from build123d import *

# Parameters (mm, degrees)
BOSS_EXTRUDE1_DEPTH   = 15
CUT_EXTRUDE1_DEPTH    = 30
SKETCH5_W             = 14
SKETCH5_H             = 36
CUT_EXTRUDE2_DEPTH    = 3
SKETCH7_R             = 1.5
CUT_EXTRUDE3_DEPTH    = 90
MIRROR1_START         = -4
MIRROR1_DEPTH         = 9
MIRROR1_START_2       = 56
MIRROR1_2_OUTLINE_W   = 60
MIRROR1_2_OUTLINE_H   = 30
MIRROR1_2_OUTLINE_W_2 = 36
MIRROR1_2_OUTLINE_H_2 = 14
MIRROR1_2_DEPTH       = 3
MIRROR1_START_3       = 59
MIRROR1_3_OUTLINE_W   = 36
MIRROR1_3_OUTLINE_H   = 14
MIRROR1_3_DEPTH       = 2
MIRROR1_4_DEPTH       = 9
MIRROR1_START_4       = 51
MIRROR1_5_DEPTH       = 4.358898944
MIRROR1_START_5       = 22.5000001
MIRROR1_6_DEPTH       = 28.4999999
MIRROR1_START_6       = -15
MIRROR1_7_OUTLINE_W   = 2
MIRROR1_7_OUTLINE_H   = 2
MIRROR1_7_DEPTH       = 30
MIRROR1_8_OUTLINE_W   = 2
MIRROR1_8_OUTLINE_H   = 36
MIRROR1_8_DEPTH       = 8
MIRROR1_START_7       = 7
MIRROR1_9_OUTLINE_W   = 2
MIRROR1_9_OUTLINE_H   = 36
MIRROR1_9_DEPTH       = 8
MIRROR1_START_8       = -6
MIRROR1_10_OUTLINE_R  = 1.5
MIRROR1_10_DEPTH      = 3
CUT_EXTRUDE5_START    = -70
CUT_EXTRUDE5_DEPTH    = 70
BOSS_EXTRUDE2_START   = -28
BOSS_EXTRUDE2_DEPTH   = 26
FILLET1_R             = 10
FILLET2_R             = 4
FILLET3_R             = 3
SKETCH9_R             = 6
CUT_EXTRUDE6_DEPTH    = 83


with BuildPart() as part:
    # Sketch1 → Boss-Extrude1 (new, symmetric)
    with BuildSketch(Plane.XY):
        with BuildLine():
            Line((5, 0), (60, 0))
            Line((60, 0), (60, -5))
            Line((60, -5), (5, -5))
            ThreePointArc((5, -5), (-2.071067812, -2.071067812), (-5, 5))
            Line((-5, 5), (-5, 60))
            Line((-5, 60), (0, 60))
            Line((0, 60), (0, 5))
            ThreePointArc((0, 5), (1.464466094, 1.464466094), (5, 0))
        make_face()
    extrude(amount=BOSS_EXTRUDE1_DEPTH, both=True)

    # Cut-Sweep1: sweep along a path in Sketch3
    with BuildLine(Plane(origin=(0, 0, 0), x_dir=(1, 0, 0), z_dir=(0, 1, 0))) as cut_sweep1_path:
        Line((60, 0), (5, 0))
    # Sketch2 → Cut-Sweep1 (sweep, cut)
    with BuildSketch(Plane(origin=(60, 0, 0), x_dir=(0, 0, -1), z_dir=(1, 0, 0))):
        Polygon((-11.5, 0), (-11.5, -1), (-13, -1), (-13, -4), (13, -4), (13, -1), (11.5, -1), (11.5, 0), align=None)
    sweep(path=cut_sweep1_path.line, mode=Mode.SUBTRACT)

    # Sketch4 → Cut-Extrude1 (cut)
    with BuildSketch(Plane(origin=(0, 0, 0), x_dir=(0, 0, -1), z_dir=(1, 0, 0))):
        with BuildLine():
            Line((1.5, 55), (1.5, 25))
            ThreePointArc((1.5, 25), (0, 23.5), (-1.5, 25))
            Line((-1.5, 25), (-1.5, 55))
            ThreePointArc((-1.5, 55), (0, 56.5), (1.5, 55))
        make_face()
    extrude(amount=-CUT_EXTRUDE1_DEPTH, mode=Mode.SUBTRACT)

    # Sketch5 → Cut-Extrude2 (cut)
    with BuildSketch(Plane(origin=(0, 0, 0), x_dir=(0, 0, -1), z_dir=(1, 0, 0))):
        with Locations((0, 40)):
            Rectangle(SKETCH5_W, SKETCH5_H)
    extrude(amount=-CUT_EXTRUDE2_DEPTH, mode=Mode.SUBTRACT)

    # Sketch7 → Cut-Extrude3 (cut, through all)
    with BuildSketch(Plane(origin=(0, -4, 0), x_dir=(1, 0, 0), z_dir=(0, 1, 0))):
        with Locations(Location((35, 7, 0), (0, 0, 270))):
            Circle(SKETCH7_R)
        with Locations(Location((35, -7, 0), (0, 0, 270))):
            Circle(SKETCH7_R)
    extrude(amount=-CUT_EXTRUDE3_DEPTH, mode=Mode.SUBTRACT)

    # Mirror1: read off the stored shape, not the designer's step
    # Mirror1 outline → Mirror1 (cut)
    with BuildSketch(Plane.YZ.offset(MIRROR1_START)):
        Polygon((0, -11.5), (0, 11.5), (-1, 11.5), (-1, 13), (-4, 13), (-4, -13), (-1, -13), (-1, -11.5), align=None)
    extrude(amount=MIRROR1_DEPTH, mode=Mode.SUBTRACT)

    # Mirror1 2 outline → Mirror1 2 (add)
    with BuildSketch(Plane.YZ.offset(MIRROR1_START_2)):
        with Locations((30, 0)):
            Rectangle(MIRROR1_2_OUTLINE_W, MIRROR1_2_OUTLINE_H)
        with Locations((40, 0)):
            Rectangle(MIRROR1_2_OUTLINE_W_2, MIRROR1_2_OUTLINE_H_2, mode=Mode.SUBTRACT)
    extrude(amount=MIRROR1_2_DEPTH)

    # Mirror1 3 outline → Mirror1 3 (add)
    with BuildSketch(Plane.YZ.offset(MIRROR1_START_3)):
        with Locations((40, 0)):
            Rectangle(MIRROR1_3_OUTLINE_W, MIRROR1_3_OUTLINE_H)
        with BuildLine():
            Line((25, 1.5), (55, 1.5))
            ThreePointArc((55, 1.5), (56.5, 0), (55, -1.5))
            Line((55, -1.5), (25, -1.5))
            ThreePointArc((25, -1.5), (23.5, 0), (25, 1.5))
        make_face(mode=Mode.SUBTRACT)
    extrude(amount=MIRROR1_3_DEPTH)

    # Mirror1 4 outline → Mirror1 4 (add)
    with BuildSketch(Plane.YZ.offset(MIRROR1_START)):
        Polygon((-1, 11.5), (0, 11.5), (0, 15), (-5, 15), (-5, -15), (0, -15), (0, -11.5), (-1, -11.5), (-1, -13), (-4, -13), (-4, 13), (-1, 13), align=None)
    extrude(amount=MIRROR1_4_DEPTH)

    # Mirror1 5 outline → Mirror1 5 (add)
    with BuildSketch(Plane.YZ.offset(MIRROR1_START_4)):
        Polygon((0, -11.5), (0, 11.5), (-1, 11.5), (-1, 13), (-4, 13), (-4, -13), (-1, -13), (-1, -11.5), align=None)
    extrude(amount=MIRROR1_5_DEPTH)

    # Mirror1 6 outline → Mirror1 6 (add)
    with BuildSketch(Plane.YZ.offset(MIRROR1_START_5)):
        Polygon((-1, 11.5), (0, 11.5), (0, 15), (-5, 15), (-5, -15), (0, -15), (0, -11.5), (-1, -11.5), (-1, -13), (-4, -13), (-4, 13), (-1, 13), align=None)
    extrude(amount=MIRROR1_6_DEPTH)

    # Mirror1 7 outline → Mirror1 7 (add)
    with BuildSketch(Plane.XY.offset(MIRROR1_START_6)):
        with BuildLine():
            Line((56, 0), (56, 5))
            ThreePointArc((56, 5), (54.535533906, 1.464466094), (51, 0))
            Line((51, 0), (55.358898944, 0))
            Line((55.358898944, 0), (55.358898944, -4))
            ThreePointArc((55.358898944, -4), (59.473163206, -0.310885546), (61, 5))
            Line((61, 5), (61, 22))
            Line((61, 22), (59, 22))
            Line((59, 22), (59, 0))
            Line((59, 0), (56, 0))
        make_face()
        with Locations((60, 59)):
            Rectangle(MIRROR1_7_OUTLINE_W, MIRROR1_7_OUTLINE_H)
    extrude(amount=MIRROR1_7_DEPTH)

    # Mirror1 8 outline → Mirror1 8 (add)
    with BuildSketch(Plane.XY.offset(MIRROR1_START_6)):
        with Locations((60, 40)):
            Rectangle(MIRROR1_8_OUTLINE_W, MIRROR1_8_OUTLINE_H)
    extrude(amount=MIRROR1_8_DEPTH)

    # Mirror1 9 outline → Mirror1 9 (add)
    with BuildSketch(Plane.XY.offset(MIRROR1_START_7)):
        with Locations((60, 40)):
            Rectangle(MIRROR1_9_OUTLINE_W, MIRROR1_9_OUTLINE_H)
    extrude(amount=MIRROR1_9_DEPTH)

    # Mirror1 10 outline → Mirror1 10 (cut)
    with BuildSketch(Plane(origin=(0, 0, 0), x_dir=(1, 0, 0), z_dir=(0, 1, 0)).offset(MIRROR1_START_8)):
        with Locations((21, -7)):
            Circle(MIRROR1_10_OUTLINE_R)
        with Locations((21, 7)):
            Circle(MIRROR1_10_OUTLINE_R)
    extrude(amount=MIRROR1_10_DEPTH, mode=Mode.SUBTRACT)

    # Sketch8 → Cut-Extrude5 (cut)
    with BuildSketch(Plane.XY.offset(15).offset(CUT_EXTRUDE5_START)):
        with BuildLine():
            Line((65.755683461, 5), (61, 5))
            ThreePointArc((61, 5), (60.659258263, 2.411809549), (59.660254038, 0))
            Line((59.660254038, 0), (60, 0))
            Line((60, 0), (60, -5))
            Line((60, -5), (51, -5))
            Line((51, -5), (51, -9.755683461))
            ThreePointArc((51, -9.755683461), (61.433843836, -5.433843836), (65.755683461, 5))
        make_face()
        with BuildLine():
            ThreePointArc((59.660254038, 0), (56, -3.660254038), (51, -5))
            Line((51, -5), (60, -5))
            Line((60, -5), (60, 0))
            Line((60, 0), (59.660254038, 0))
        make_face()
        with BuildLine():
            Line((-4, -5), (5, -5))
            ThreePointArc((5, -5), (0, -3.660254038), (-3.660254038, 0))
            Line((-3.660254038, 0), (-4, 0))
            Line((-4, 0), (-4, -5))
        make_face()
    extrude(amount=CUT_EXTRUDE5_DEPTH, mode=Mode.SUBTRACT)

    # Sketch8<3> → Boss-Extrude2 (add)
    with BuildSketch(Plane.XY.offset(15).offset(BOSS_EXTRUDE2_START)):
        with BuildLine():
            ThreePointArc((-3.660254038, 0), (0, -3.660254038), (5, -5))
            Line((5, -5), (5, 0))
            ThreePointArc((5, 0), (1.464466094, 1.464466094), (0, 5))
            Line((0, 5), (-5, 5))
            ThreePointArc((-5, 5), (-4.659258263, 2.411809549), (-3.660254038, 0))
        make_face()
    extrude(amount=BOSS_EXTRUDE2_DEPTH)

    # Fillet1
    fillet1_edges = [part.edges().sort_by_distance(p)[0] for p in [
        (58.5, 60, -15),
        (58.5, 60, 15),
        (-2.5, 60, 15),
        (-2.5, 60, -15),
    ]]
    fillet(fillet1_edges, radius=FILLET1_R)

    # Fillet2
    fillet2_edges = [part.edges().sort_by_distance(p)[0] for p in [
        (57.5, 58, 7),
        (57.5, 58, -7),
        (-1.5, 58, 7),
        (-1.5, 58, -7),
    ]]
    fillet(fillet2_edges, radius=FILLET2_R)

    # Fillet3
    fillet3_edges = [part.edges().sort_by_distance(p)[0] for p in [
        (28, -4, 13),
        (28, -4, -13),
    ]]
    fillet(fillet3_edges, radius=FILLET3_R - 0.0001)  # a hair under: the kernel refuses the full size

    # Sketch9 → Cut-Extrude6 (cut)
    with BuildSketch(Plane.ZY.offset(5)):
        with Locations((0, 13)):
            Circle(SKETCH9_R)
    extrude(amount=-CUT_EXTRUDE6_DEPTH, mode=Mode.SUBTRACT)


solid = part.part
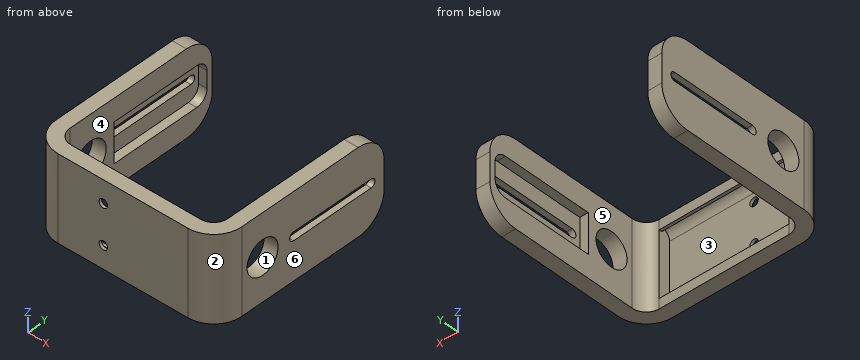
Source: CAD feature listing. Evaluate the final solid. Frame: model axes, mm. Face numbers are marked on the shaded views. A direction names the side the tool comes from. Round coordinates to 2 decimals unless told otherwise and drop trailing zeros. Loops run counter-clockwise (first coordinate to the right, second up) from the corner with the lowest first, then second, coordinate; pieces in that order, holes last. Notation, with made-up numbers: (52, 0) - (86, 0) arc R27 ccw to (86, 35) - close; hole circle Ø2 at (1, -9). An arc over 180 degrees is marked (long way). Write item = value, one per line. Start each with the question number.
(1) Ray query, line 1 along X through (y, z) = (11, 14); line 2 along Y through (x, z) = (-2.6, 0); line 3 along Y through (x, z) = (-0.5, -3). Return the intervals inside material, ascending. Write a range as from..to.
(2) Set-up query: the marked faces 5 and 6. Return all of +Z, -Z, +X, -X, +Y, -Y with unobstructed straight access to the full face (end or side cutting, diameter ignored); none if empty.
(3) Pull-direction query (Y, two-part tool) for the marked faces 1, 2, 3 and 4; classes: +Y half, -Y half, draft (parallel to the pull), parting line (faces both ways), or undercut.
(4) Section query A-A, the plane x = 21. State how many separate pieces and enclosed holes the cut face has, plus the area to 3 significant figures.
(5) Section query B-B, the plane y = 33. Output: boundary loops of the cut face in (x, z), plus the area to 3 significant figures.
(6) Section query D-D, the plane y = 1.5. Output: boundary loops of the cut face in (x, z), plus the area to 3 significant figures.
(7) Pin query (flat end, axial travel): pin 1 (1.5 mm diameter, centred on x = 58, z = -0.5, fed in from -Y); pin 2 (8 mm diameter, centred on x = 34.5, z = -8.5, fed in from +Y); pin 3 (7 mm diameter, centred on y = 13, z = 0, fed in from +X); pin 4 (1.5 mm diameter, centred on x = 8.5, z = 5, fed in from +Y). Return the tip coordinate at first contact, or that it passes through.
Conclusion:
q1.line_1 = -5..0, 56..61
q1.line_2 = -1.5..7, 19..22, 58..60
q1.line_3 = -3.35..7.8, 18.2..22, 58..60
q2.face_5 = +Z, -Z, +Y
q2.face_6 = +Z, -Z, +X, +Y, -Y
q3.face_1 = undercut
q3.face_2 = -Y half
q3.face_3 = +Y half
q3.face_4 = draft
q4.separate_pieces = 3
q4.enclosed_holes = 0
q4.area = 46.9 mm2
q5.outline = (-5, -15) - (0, -15) - (0, -7) - (-3, -7) - (-3, -1.5) - (-5, -1.5) - close; (-5, 1.5) - (-3, 1.5) - (-3, 7) - (0, 7) - (0, 15) - (-5, 15) - close; (56, -15) - (61, -15) - (61, -1.5) - (59, -1.5) - (59, -7) - (56, -7) - close; (56, 7) - (59, 7) - (59, 1.5) - (61, 1.5) - (61, 15) - (56, 15) - close
q5.area = 204 mm2
q6.outline = (-4.37, -15) - (1.43, -15) - (1.43, 15) - (-4.37, 15) - close; (54.57, -15) - (60.37, -15) - (60.37, 15) - (54.57, 15) - close
q6.area = 348 mm2
q7.pin_1 = -2.81
q7.pin_2 = 0
q7.pin_3 = through
q7.pin_4 = -4
